Input: part model. Units: mm. Frame: model coordinates. Face numbers are marked on the shaded views. A direction names the side the tool comes from. Give positions to 0.01 mm unless a question says otherwise; leave off trailing zeros. Loops run counter-clockwise (first coordinate to the right, second up) from the corner with the lowest first, then second, coordinate; pieces in that order, holes last. Notation, with made-up numbers: (82.5, -32) -> (112.5, -32) arc R20 ccw to (112.5, -20) -> close; hole circle Ø1 at (41, -8.5). An arc over 180 degrees is marked (long way). Use CSV: the item, a comma, the result in double quotes.
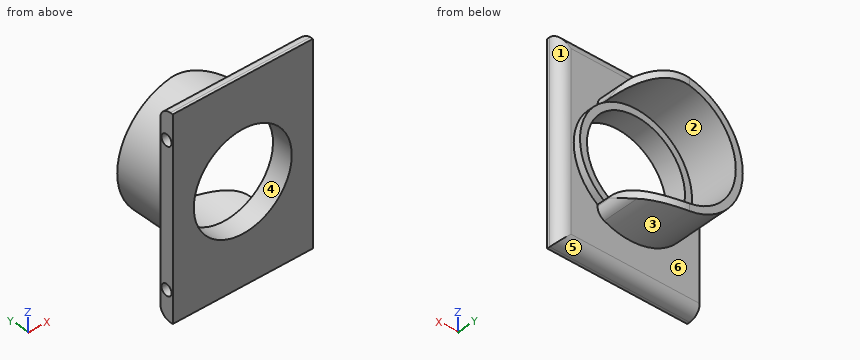
```python
from build123d import *

# Parameters (mm, degrees)
CROQUIS3_W                 = 300
CROQUIS3_H                 = 140
SALIENTE_EXTRUIR1_DEPTH    = 10
CROQUIS5_R                 = 40
CROQUIS5_R_2               = 35
SALIENTE_EXTRUIR2_DEPTH    = 5
SALIENTE_EXTRUIR5_DEPTH    = 40
REDONDEO3_START            = -46
REDONDEO3_DEPTH            = 13.273863656
REDONDEO4_START            = -44.452221542
REDONDEO4_DEPTH            = 90.452221542
CORTAR_EXTRUIR1_START      = -40
CROQUIS7_R                 = 35
CORTAR_EXTRUIR1_DEPTH      = 40
MATRIZL1_COUNT             = 3
MATRIZL1_PITCH             = 100
CORTAR_EXTRUIR3_DEPTH      = 171.293863683
CORTAR_EXTRUIR3_DEPTH_BACK = 171.293863683
CROQUIS10_W                = 200
CROQUIS10_H                = 140
CROQUIS12_R                = 4
CORTAR_EXTRUIR4_DEPTH      = 30
REDONDEO5_R                = 8


with BuildPart() as part:
    # Croquis3 → Saliente-Extruir1 (new body)
    with BuildSketch(Plane(origin=(0, 0, 0), x_dir=(1, 0, 0), z_dir=(0, 1, 0))):
        Rectangle(CROQUIS3_W, CROQUIS3_H)
    extrude(amount=SALIENTE_EXTRUIR1_DEPTH)

    # Croquis5 → Saliente-Extruir2 (add)
    # profile 1 of 3: a face of its own
    with BuildSketch(Plane(origin=(0, 10, 0), x_dir=(1, 0, 0), z_dir=(0, 1, 0))):
        with Locations(Location((-100, 0, 0), (0, 0, 270))):
            Circle(CROQUIS5_R)
        with Locations(Location((-100, 0, 0), (0, 0, 270))):
            Circle(CROQUIS5_R_2, mode=Mode.SUBTRACT)
    # profile 2 of 3: a face of its own
    with BuildSketch(Plane(origin=(0, 10, 0), x_dir=(1, 0, 0), z_dir=(0, 1, 0))):
        with Locations(Location((0, 0, 0), (0, 0, 270))):
            Circle(CROQUIS5_R)
        with Locations(Location((0, 0, 0), (0, 0, 270))):
            Circle(CROQUIS5_R_2, mode=Mode.SUBTRACT)
    # profile 3 of 3: a face of its own
    with BuildSketch(Plane(origin=(0, 10, 0), x_dir=(1, 0, 0), z_dir=(0, 1, 0))):
        with Locations(Location((100, 0, 0), (0, 0, 270))):
            Circle(CROQUIS5_R)
        with Locations(Location((100, 0, 0), (0, 0, 270))):
            Circle(CROQUIS5_R_2, mode=Mode.SUBTRACT)
    extrude(amount=SALIENTE_EXTRUIR2_DEPTH)

    # Croquis6 → Saliente-Extruir5 (add)
    with BuildSketch(Plane(origin=(0, 10, 0), x_dir=(1, 0, 0), z_dir=(0, 1, 0))):
        with BuildLine():
            Line((-77, 33.823069051), (-77, 32.726136344))
            ThreePointArc((-77, 32.726136344), (-140, 0), (-77, -32.726136344))
            Line((-77, -32.726136344), (-77, -33.823069051))
            ThreePointArc((-77, -33.823069051), (-78.293810846, -38.185067105), (-81.756756757, -41.136165062))
            ThreePointArc((-81.756756757, -41.136165062), (-145, 0), (-81.756756757, 41.136165062))
            ThreePointArc((-81.756756757, 41.136165062), (-78.293810846, 38.185067105), (-77, 33.823069051))
        make_face()
    saliente_extruir5 = extrude(amount=SALIENTE_EXTRUIR5_DEPTH)

    # Redondeo3: read off the stored shape, not the designer's step
    # Redondeo3 outline → Redondeo3 (cut)
    with BuildSketch(Plane.XY.offset(REDONDEO3_START)):
        with BuildLine():
            ThreePointArc((-107.000000862, 50), (-85.786796869, 41.21320374), (-77, 20))
            Line((-77, 20), (-77, 50))
            Line((-77, 50), (-107.000000862, 50))
        make_face()
    redondeo3 = extrude(amount=REDONDEO3_DEPTH, mode=Mode.SUBTRACT)

    # Redondeo4: read off the stored shape, not the designer's step
    # Redondeo4 outline → Redondeo4 (cut)
    with BuildSketch(Plane.XY.offset(REDONDEO4_START)):
        with BuildLine():
            ThreePointArc((-107.000000862, 50), (-85.786796869, 41.21320374), (-77, 20))
            Line((-77, 20), (-77, 50))
            Line((-77, 50), (-107.000000862, 50))
        make_face()
    redondeo4 = extrude(amount=REDONDEO4_DEPTH, mode=Mode.SUBTRACT)

    # Croquis7 → Cortar-Extruir1 (cut)
    with BuildSketch(Plane(origin=(0, 10, 0), x_dir=(1, 0, 0), z_dir=(0, 1, 0)).offset(CORTAR_EXTRUIR1_START)):
        with Locations(Location((-100, 0, 0), (0, 0, 270))):
            Circle(CROQUIS7_R)
    cortar_extruir1 = extrude(amount=CORTAR_EXTRUIR1_DEPTH, mode=Mode.SUBTRACT)

    # MatrizL1: Saliente-Extruir5, Redondeo3, Redondeo4, Cortar-Extruir1 ×3
    with Locations(*[(i * MATRIZL1_PITCH, 0, 0) for i in range(1, MATRIZL1_COUNT)]):
        add(saliente_extruir5)
        add(redondeo3, mode=Mode.SUBTRACT)
        add(redondeo4, mode=Mode.SUBTRACT)
        add(cortar_extruir1, mode=Mode.SUBTRACT)

    # Croquis10 → Cortar-Extruir3 (cut, two sides: drawn at the far end of the back side and taken through both)
    with BuildSketch(Plane(origin=(0, 10, 0), x_dir=(1, 0, 0), z_dir=(0, 1, 0)).offset(-CORTAR_EXTRUIR3_DEPTH_BACK)):
        with Locations((50, 0)):
            Rectangle(CROQUIS10_W, CROQUIS10_H)
    extrude(amount=CORTAR_EXTRUIR3_DEPTH + CORTAR_EXTRUIR3_DEPTH_BACK, mode=Mode.SUBTRACT)

    # Croquis12 → Cortar-Extruir4 (cut)
    with BuildSketch(Plane.ZY.offset(150)):
        with Locations((-50, 5)):
            Circle(CROQUIS12_R)
        with Locations((50, 5)):
            Circle(CROQUIS12_R)
    extrude(amount=-CORTAR_EXTRUIR4_DEPTH, mode=Mode.SUBTRACT)

    # Redondeo5
    redondeo5_edges = [part.edges().sort_by_distance(p)[0] for p in [
        (-100, 10, -70),
        (-50, 10, 0),
        (-100, 10, 70),
    ]]
    fillet(redondeo5_edges, radius=REDONDEO5_R)


solid = part.part
```
1) Mould query, pull axis Z, two halves, no side actions, for the marked faces 1, 2, 3 and 4. Classes: pulls with the +Z half, pulls with the -Z half, needs draft (parallel to the pull), parting line crosses it, or undercut.
From the geometry:
face 1,"needs draft"
face 2,"undercut"
face 3,"parting line crosses it"
face 4,"undercut"
2) Ray query, line 1 (Y direction, x = -131.25, z = -50); line 2 (Y direction, x = -132.5, z = -39); line 3 (Z direction, x = -131, y = 38.5). Return the intervals inside material, ascending.
From the geometry:
line 1,"y = 0 to 1, 9 to 10"
line 2,"y = 0 to 10"
line 3,"z = -32.62 to -25.28, 25.28 to 32.62"
3) Section query A-A (y = 12.5). Return loops of the section in (x, z).
From the geometry:
outline,"(-81.76, -41.14) arc R8 ccw to (-77, -33.82) -> (-77, -32.73) arc R40 ccw to (-77, 32.73) -> (-77, 33.82) arc R8 ccw to (-81.76, 41.14) arc R45 ccw (long way) to start; hole circle Ø70 at (-100, 0)"
4) Section query D-D (x = -100). Return loops of the section in (y, z).
From the geometry:
outline,"(0, -70) -> (2, -70) arc R8 ccw to (10, -62) -> (10, -45) -> (49.17, -45) -> (49.17, -40) -> (15, -40) -> (15, -35) -> (0, -35) -> close; (0, 35) -> (15, 35) -> (15, 40) -> (49.17, 40) -> (49.17, 45) -> (10, 45) -> (10, 62) arc R8 ccw to (2, 70) -> (0, 70) -> close"
5) Contact query for flat-ended pins moving along their axis: pin 1 (12 mm diameter, centred on x = -87, y = 38.5, fed in from +Z); pin 2 (1.2 mm diameter, centred on y = 17.5, z = 33.5, fed in from +X); pin 3 (1.5 mm diameter, centred on y = 32.5, z = 41.5, fed in from +X). Output: stop coordinate, or through.
From the geometry:
pin 1,"stops at z = 44.45"
pin 2,"stops at x = -77"
pin 3,"stops at x = -81"
6) Section query C-C (x = -131.5). Return loops of the section in (y, z).
From the geometry:
outline,"(0, -70) -> (2, -70) arc R8 ccw to (10, -62) -> (10, -32.14) -> (50, -32.14) -> (50, -24.65) -> (15, -24.65) -> (15, -15.26) -> (0, -15.26) -> close; (0, 15.26) -> (15, 15.26) -> (15, 24.65) -> (50, 24.65) -> (50, 32.14) -> (10, 32.14) -> (10, 62) arc R8 ccw to (2, 70) -> (0, 70) -> close; hole circle Ø8 at (5, -50); hole circle Ø8 at (5, 50)"
7) Section query B-B (z = -11). Return loops of the section in (x, y).
From the geometry:
outline,"(-150, 0) -> (-133.23, 0) -> (-133.23, 15) -> (-138.46, 15) -> (-138.46, 50) -> (-143.63, 50) -> (-143.63, 10) -> (-150, 10) -> close; (-66.77, 0) -> (-50, 0) -> (-50, 2) arc R8 ccw to (-58, 10) -> (-61.54, 10) -> (-61.54, 15) -> (-66.77, 15) -> close"
8) Reachability of the marked faces 5 and 6 from +Z, -Z, +X, -X, +Y, -Y: full face, straight path, thin tool, end or side. Return the list, or none.
From the geometry:
face 5,"-Z, +X, -X, +Y"
face 6,"+Y"
